Autodesk Inventor part; units mm, degrees
ref_plane "Начальная плоскость" through (0, 0, -40) normal (0, 0, 1) x (1, 0, 0)
ref_plane "Конечная плоскость" through (0, 0, 469.1169) normal (0, 0, 1) x (1, 0, 0)
ref_plane "РабПлоскость4" through (21.07, 40, 469.1169) normal (0, -0.3827, 0.9239) x (1, 0, 0)
ref_plane "Начальная плоскость" through (0, 0, -40) normal (0, 0, 1) x (1, 0, 0)
ref_plane "Конечная плоскость" through (0, 0, 469.1169) normal (0, 0, 1) x (1, 0, 0)
sketch "Эскиз" plane through (0, 0, 0) normal (0, 0, 1) x (1, 0, 0)
  line L0 (-1.43, 0) -> (-1.43, 40)
  line L1 (-1.43, 40) -> (43.57, 40)
  line L2 (43.57, 40) -> (43.57, 38.1774)
  line L3 (39.9881, 34.1993) -> (11.2338, 31.1771)
  line L4 (4.07, 23.221) -> (4.07, 0)
  line L5 (4.07, 0) -> (-1.43, 0) construction
  line L6 (23.82, 40) -> (23.82, 32.5) construction
  line L7 (43.57, 34.5758) -> (43.57, 32.5) construction
  line L8 (43.57, 32.5) -> (23.82, 32.5) construction
  line L9 (0, 15) -> (0, -27) construction
  line L10 (-5.539, 0) -> (16.0067, 0) construction
  line L11 (-1.43, 0) -> (-1.43, -40)
  line L12 (-1.43, -40) -> (43.57, -40)
  line L13 (43.57, -40) -> (43.57, -38.1774)
  line L14 (39.9881, -34.1993) -> (11.2338, -31.1771)
  line L15 (4.07, -23.221) -> (4.07, 0)
  arc A0 (11.2338, 31.1771) -> (4.07, 23.221) centre (12.07, 23.221) ccw
  arc A1 (4.07, -23.221) -> (11.2338, -31.1771) centre (12.07, -23.221) ccw
  arc A2 (39.9881, 34.1993) -> (43.57, 38.1774) centre (39.57, 38.1774) ccw
  arc A3 (43.57, -38.1774) -> (39.9881, -34.1993) centre (39.57, -38.1774) ccw
  line L16 (0, 56) -> (0, -56) construction
  line L17 (-15.5135, 0) -> (54.308, 0) construction
  point P0 (4.07, 30.4242)
  point P1 (43.57, -34.5758)
  point P2 (4.07, -30.4242)
  point P3 (23.82, -40)
  point P4 (23.82, -32.5)
  dimension "d0" = 5.5
  dimension "d1" = 40
  dimension "d2" = 45
  dimension "d3" = 7.5
  dimension "d4" = 19.75
  dimension "d5" = 2.0758
  dimension "d23" = 8
  dimension "d24" = 4
  dimension "d25" = 1.43
extrude "Тело" add sketch "Эскиз" along normal up to surface (509.1169 mm away) from surface at -40
sketch "Sketch3" plane through (0, 0, 0) normal (0, 0, 1) x (1, 0, 0)
  line L0 (0, 0) -> (10, 0)
ref_plane "Work Plane3" through (0, 0, 0) normal (0, -1, 0) x (1, 0, 0)
sketch "Sketch4" plane through (0, 0, 0) normal (0, -1, 0) x (1, 0, 0)
  line L0 (-2, -40) -> (12, -40)
  line L1 (-2, 469.1169) -> (12, 469.1169)
  dimension "d29" = 509.1169
ref_plane "РабПлоскость4" through (21.07, 40, 469.1169) normal (0, -0.3827, 0.9239) x (1, 0, 0)
split "Разделение1" plane through (21.07, 40, 469.1169) removes the side toward (0, -0.3827, 0.9239)
ref_plane "РабПлоскость8" through (753.131, -459.0658, 459.0658) normal (0, -0.7071, -0.7071) x (1, 0, 0)
split "Разделение2" plane through (753.131, -459.0658, 459.0658) removes the side toward (0, -0.7071, -0.7071)
equation "\"d0\" = G_T"
equation "\"d1\" = 0.5 * G_H"
equation "\"d2\" = G_W"
equation "\"d3\" = G_T1"
equation "\"d4\" = G_C"
equation "\"d23\" = G_IR"
equation "\"d24\" = G_ER"
equation "\"d25\" = ex"
equation "\"d6\" = G_L"
equation "\"G_W\" = 45"
equation "\"G_T\" = 5.5"
equation "\"G_T1\" = 7.5"
equation "\"G_NG\" = 0.105104"
equation "\"G_ER\" = 4"
equation "\"G_IR\" = 8"
equation "\"G_C\" = 19.75"
equation "\"G_L\" = d29"
equation "\"ex\" = 1.43"
equation "\"G_OFFSET_END\" = 16.56854"
equation "\"d27\" = G_OFFSET_END + B_L"
equation "\"B_L\" = 452.54834"
properties part number "ISO 657/11 - CH 80 x 8 - 509,12" material "Сталь, мягкая"
Geometry: final body of the model. Coordinates: model frame, mm. A direction names the side the tool comes from. Coordinates: 2 decimals unless noted, no trailing zeros. Loops run counter-clockwise (first coordinate to the right, second up) from the corner with the lowest first, then second, coordinate; pieces in that order, holes last. Notation, with made-up numbers: (75, 30.25) - (125, 30.25) arc R24 ccw to (125, 62.25) - close; hole circle Ø6 at (68.25, 77.5). An arc over 180 degrees is marked (long way). Put each result on its own line as item: value. Start each with the question number.
Q1. Set-up query: faces 1 (the cylindrical face through (6.07, 28.51, 213.67)), 2 (the flat face through (3, 0, 0)). Return all of +Z, -Z, +X, -X, +Y, -Y with unobstructed straight access to the full face (end or side cutting, diameter ignored); none if empty.
Q2. Cut plane B-B, the plane z = 145. Return loops of the section in (x, y), and give its area (3 significant figures).
Q3. Cut plane C-C, the plane y = 10. Return loops of the section in (x, z), and give its area (3 significant figures).
Q4. Pull-direction query (Y, two-part tool) for faces 3 (the flat face through (2.63, -0.19, 452.47)), 4 (the flat face through (-1.43, -1, 211)), 5 (the flat face through (25.81, 32.71, 212.75)); classes: released by +Y, released by -Y, zero draft, split by the parting line, or undercut.
Q5. Line query: line 1 (X direction, y = 3, z = 131); line 2 (Y direction, x = 7.5, z = 236.5); line 3 (Y direction, x = 24, z = 324). Output: solid intervals per line, ascending.
Q6. Cut plane A-A, the plane x = 17. Return loops of the section in (y, z).
Q7. Pin query (flat end, axial travel): pin 1 Ø2 at (x, y) = (8.5, -30.5) entering from -Z; pin 2 Ø8 at (x, z) = (6, 16.5) entering from -Y. Return the tip coordinate at first contact, or that it passes through.
Filled sheet:
1. face 1: +Z, -Z, +X
1. face 2: -Z, +X, -X, -Y
2. outline: (-1.43, -40) - (43.57, -40) - (43.57, -38.18) arc R4 ccw to (39.99, -34.2) - (11.23, -31.18) arc R8 cw to (4.07, -23.22) - (4.07, 23.22) arc R8 cw to (11.23, 31.18) - (39.99, 34.2) arc R4 ccw to (43.57, 38.18) - (43.57, 40) - (-1.43, 40) - close
2. area: 1,050 mm²
3. outline: (-1.43, -10) - (4.07, -10) - (4.07, 456.69) - (-1.43, 456.69) - close
3. area: 2,570 mm²
4. face 3: released by -Y
4. face 4: zero draft
4. face 5: undercut
5. line 1: -1.43 to 4.07
5. line 2: -40 to -29.79, 29.79 to 40
5. line 3: -40 to -32.52, 32.52 to 40
6. outline: (-40, 40) - (-31.78, 31.78) - (-31.78, 439.38) - (-40, 435.98) - close; (31.78, -31.78) - (40, -40) - (40, 469.12) - (31.78, 465.71) - close
7. pin 1: z = 29.91
7. pin 2: y = -20
